Autodesk Inventor part; units mm, degrees
ref_plane "YZ Plane" through (0, 0, 0) normal (1, 0, 0) x (0, 1, 0)
ref_plane "XZ Plane" through (0, 0, 0) normal (0, 1, 0) x (-1, 0, 0)
ref_plane "XY Plane" through (0, 0, 0) normal (0, 0, 1) x (1, 0, 0)
sketch "Sketch1" plane through (0, 0, 0) normal (0, 1, 0) x (-1, 0, 0)
  line L0 (0, 0) -> (150, 0)
  line L1 (150, 0) -> (150, -10)
  line L2 (150, -10) -> (0, -10)
  line L3 (0, -10) -> (0, 0)
  dimension "d0" = 150
  dimension "d1" = 10
extrude "Extrusion1" add sketch "Sketch1" along normal blind 70
sketch "Sketch2" plane through (-150, 0, 0) normal (0, 0, 1) x (1, 0, 0)
  line L0 (0, 70) -> (150, 70)
  line L1 (150, 0) -> (0, 0)
  line L2 (0, 0) -> (0, 70)
  point P0 (75, 55)
  dimension "d5" = 55
  dimension "d6" = 75
hole "Hole1" at (-75, 55, 0) direction (0, 0, -1) diameter 10 depth 10 tip angle 118
chamfer "Chamfer1" distance 4 angle 45 1 edges at (-75, 60, 0)
sketch "Sketch3" plane through (0, 0, 0) normal (0, -1, 0) x (1, 0, 0)
  line L0 (0, 0) -> (-150, 0)
  line L1 (-150, 0) -> (-150, -10)
  line L2 (0, -10) -> (0, 0)
  point P0 (-40, -5)
  point P1 (-110, -5)
  dimension "d18" = 5
  dimension "d19" = 5
  dimension "d20" = 40
  dimension "d21" = 40
hole "Hole2" at (-40, 0, -5) at (-110, 0, -5) direction (0, 1, 0) diameter 2.459 depth 10 tip angle 118
chamfer "Chamfer2" distance 4 angle 45 1 edges at (-75, 60, -10)
properties part number "cathetherEntry"
CAD build for the part. Positions are in the model's coordinates, mm. Give positions to 0.01 mm unless a question says otherwise; leave off trailing zeros. Write each loop counter-clockwise with the first axis right and the second up, starting at its lowest first coordinate (ties: lowest second). Pieces come first, ordered by that corner, then holes. Notation, with made-up numbers: (-1, -34) -> (25, -34) arc R31 ccw to (25, -3) -> close; hole circle Ø1 at (65, 68.25). An arc over 180 degrees is marked (long way). Return JSON: item names as keys, results as strings.
Item 1: Drill centre lines: probe 1 along X at (y, z) = (6.5, -5); probe 2 along X at (y, z) = (55, -4.9); probe 3 along Z at (x, y) = (-40, 3). Where is each one in solid material? Low to high.
Answer below:
{"probe 1": "x = -150 to -111.23, -108.77 to -41.23, -38.77 to 0", "probe 2": "x = -150 to -80, -70 to 0", "probe 3": "z = -10 to -6.23, -3.77 to 0"}
Item 2: Drop a flat-ended pin along its axis: pin 1 (11.5 mm diameter, centred on x = -75, y = 55, fed in from -Z). Give the stop position or say it passes through.
Answer below:
{"pin 1": "stops at z = -6.75"}
Item 3: Band-saw the part on A-A (x = -75). List the corners of the cut face in (y, z), then the cut area to 3 significant figures.
Answer below:
{"outline": "(0, -10) -> (46, -10) -> (50, -6) -> (50, -4) -> (46, 0) -> (0, 0) -> close; (60, -6) -> (64, -10) -> (70, -10) -> (70, 0) -> (64, 0) -> (60, -4) -> close", "area": "568 mm2"}
Item 4: Two-plate mould, pull along X, no slides. Class faces 1 (the cylindrical face through (-70.12, 56.08, -5.01)), 2 (the flat face through (-74, 35, 0)), 3 (the flat face through (0, 35, -5)), 4 (the flat face through (-150, 35, -5)): +X half, -X half, draft (parallel to the pull), parting line (faces both ways), or undercut.
Answer below:
{"face 1": "undercut", "face 2": "draft", "face 3": "+X half", "face 4": "-X half"}
Item 5: Band-saw the part on B-B (y = 55). List the corners of the cut face in (x, z), then the cut area to 3 significant figures.
Answer below:
{"outline": "(-150, -10) -> (-84, -10) -> (-80, -6) -> (-80, -4) -> (-84, 0) -> (-150, 0) -> close; (-70, -6) -> (-66, -10) -> (0, -10) -> (0, 0) -> (-66, 0) -> (-70, -4) -> close", "area": "1,370 mm2"}
